Design review of the part built by this model. Coordinates are the model's own, in mm. A direction names the side the tool comes from. Round coordinates to 2 decimals unless told otherwise and drop trailing zeros. Loops run counter-clockwise (first coordinate to the right, second up) from the corner with the lowest first, then second, coordinate; pieces in that order, holes last. Notation, with made-up numbers: M -7,25.25 L 2,25.25 A18 cw 2,49.25 Z; hole C 48.5,8.25 d1. An arc over 180 degrees is marked long. One line per item, written item: value. Start each with the question number.
Item 1: We need section A-A (z = 5.75). Write out the cut boundary in (x, y).
Item 2: Mouldability with a two-part tool opening along Y and no side actions: class faces 3 (the cylindrical face through (77.22, 10.85, 9.86)), 4 (the cylindrical face through (4.563, 4.811, 9.86)), 5 (the cylindrical face through (51.937, 16.446, 14.93)) as released by +Y, released by -Y, zero draft, split by the parting line, or undercut.
Item 3: For line 1 along Y through (x, z) = (16, 5); line 2 along Y through (x, z) = (16, 16.75); line 3 along X through (y, z) = (21, 11.25), list the stretches that pass through material, from the lowest coordinate up.
Item 4: We need section D-D (y = 30). Write out the cut boundary in (x, z), then the cut area to 3 significant figures.
Item 5: We need section B-B (x = 13). Write out the cut boundary in (y, z).
Item 6: For faces 1 (the cylindrical face through (8.898, 63.246, 9.86)), 2 (the cylindrical face through (25.593, 51.93, 14.93)), list the 3-axis set-ups (+Z, -Z, +X, -X, +Y, -Y) from which the entire face can be reached by the end or side of a thin tool; tool diameter is ignored.
Item 7: Clearance check with flat-ended pins moving along their axes: pin 1 (6 mm diameter, centred on x = 60.5, y = 21, fed in from +Z); pin 2 (2 mm diameter, centred on y = 37.5, z = 17, fed in from +X); pin 3 (1 mm diameter, centred on y = 28, z = 3.5, fed in from +X). State where each tip first meets the part, or that it passes through.
Item 8: We need section C-C (y = 46.5). Write out the cut boundary in (x, z).
from build123d import *

# Parameters (mm, degrees)
F0_R     = 10.045621
F0_R_2   = 10.145405
F0_R_3   = 10.057845
F1_DEPTH = 20
F0_R_4   = 4.017037
F0_R_5   = 4.066063
F0_R_6   = 4.025873
F2_DEPTH = 10


with BuildPart() as f1:
    # F0 (on Top) → F1 (new body)
    with BuildSketch(Plane.XY):
        with BuildLine():
            ThreePointArc((0, 16), (4.686292, 4.686292), (16, 0))
            Line((16, 0), (62.072559, 0))
            ThreePointArc((62.072559, 0), (77.309287, 11.117161), (71.37237, 29.019736))
            Line((71.37237, 29.019736), (25.299811, 61.928706))
            ThreePointArc((25.299811, 61.928706), (8.678695, 63.135653), (0, 48.908971))
            Line((0, 48.908971), (0, 16))
        make_face()
        with Locations((16, 16)):
            Circle(F0_R, mode=Mode.SUBTRACT)
        with Locations((62.072559, 16)):
            Circle(F0_R_2, mode=Mode.SUBTRACT)
        with Locations((16, 48.908971)):
            Circle(F0_R_3, mode=Mode.SUBTRACT)
    extrude(amount=F1_DEPTH)

    # F0 (on Top) → F2 (join)
    with BuildSketch(Plane.XY):
        with Locations((16, 48.908971)):
            Circle(F0_R_3)
        with Locations((16, 48.908971)):
            Circle(F0_R_4, mode=Mode.SUBTRACT)
        with Locations((16, 16)):
            Circle(F0_R)
        with Locations((16, 16)):
            Circle(F0_R_5, mode=Mode.SUBTRACT)
        with Locations((62.072559, 16)):
            Circle(F0_R_2)
        with Locations((62.072559, 16)):
            Circle(F0_R_6, mode=Mode.SUBTRACT)
    extrude(amount=F2_DEPTH)


solid = f1.part
A:
1. outline: M 0,16 A16 ccw 16,0 L 62.07,0 A16 ccw 71.37,29.02 L 25.3,61.93 A16 ccw 0,48.91 Z; hole C 16,16 d8.13; hole C 16,48.91 d8.03; hole C 62.07,16 d8.05
2. face 3: split by the parting line
2. face 4: released by -Y
2. face 5: undercut
3. line 1: 0 to 11.93, 20.07 to 44.89, 52.93 to 64.91
3. line 2: 0 to 5.95, 26.05 to 38.85, 58.97 to 64.91
3. line 3: 0 to 7.29, 24.71 to 53.24, 70.9 to 77.27
4. outline: M 0,0 L 70,0 L 70,20 L 0,20 Z
4. area: 1,400 mm2
5. outline: M 0.28,0 L 13.26,0 L 13.26,10 L 6.41,10 L 6.41,20 L 0.28,20 Z; M 18.74,0 L 46.24,0 L 46.24,10 L 39.31,10 L 39.31,20 L 25.59,20 L 25.59,10 L 18.74,10 Z; M 51.58,0 L 64.63,0 L 64.63,20 L 58.51,20 L 58.51,10 L 51.58,10 Z
6. face 1: +Z, -Z, +Y
6. face 2: +Z
7. pin 1: z = 10
7. pin 2: x = 60.9
7. pin 3: x = 73.2
8. outline: M 0,0 L 12.79,0 L 12.79,10 L 6.23,10 L 6.23,20 L 0,20 Z; M 19.21,0 L 46.9,0 L 46.9,20 L 25.77,20 L 25.77,10 L 19.21,10 Z
